Could you check a few things on this drawing? It's one solid part, dimensions in mm from its lowest x, y, z. A direction names the side the tool comes from. Round coordinates to 2 decimals unless told otherwise and drop trailing zeros. Write each loop counter-clockwise with the first axis right and the second up, starting at its lowest first coordinate (ties: lowest second). Pieces come first, ordered by that corner, then holes. Notation, with made-up numbers: (78.25, 71) - (104.25, 71) arc R33 ccw to (104.25, 105) - close; hole circle Ø5 at (-37.5, -39). An arc over 180 degrees is marked (long way). Use one line per item in the form item = value. Start each with the question number.
1. Which directions (+Z, -Z, +X, -X, +Y, -Y) give clear straight access to the entire face, cutting with the end or side of a thin tool? Please do the marked faces 4 and 5.
2. I want a section at A-A, the plane x = 10. List the corners of the cut face in (y, z) for me, plus the area to 3 significant figures.
3. We'd pull the mould along X, two halves only. Please class the marked faces 1, 2 and 3: +X half, -X half, draft (parallel to the pull), parting line (faces both ways), or undercut.
4. If I drill on line 1 along Y through (x, z) = (10, 5.75); line 2 along Z through (x, y) = (14.25, 14.5); line 3 along Y through (x, z) = (11.5, 1.25), over which ranges is the centre line in solid material (lowest first)?
5. Will this pin go through, and if not, where does the flat tip stop? pin 1 (2 mm diameter, centred on x = 7, z = 1, fed in from +Y).
6. I want a section at C-C, the plane z = 7. List the corners of the cut face in (x, y) for me, plus the area to 3 significant figures.
7. I want a section at B-B, the plane y = 4. List the corners of the cut face in (x, z) for me, plus the area to 3 significant figures.
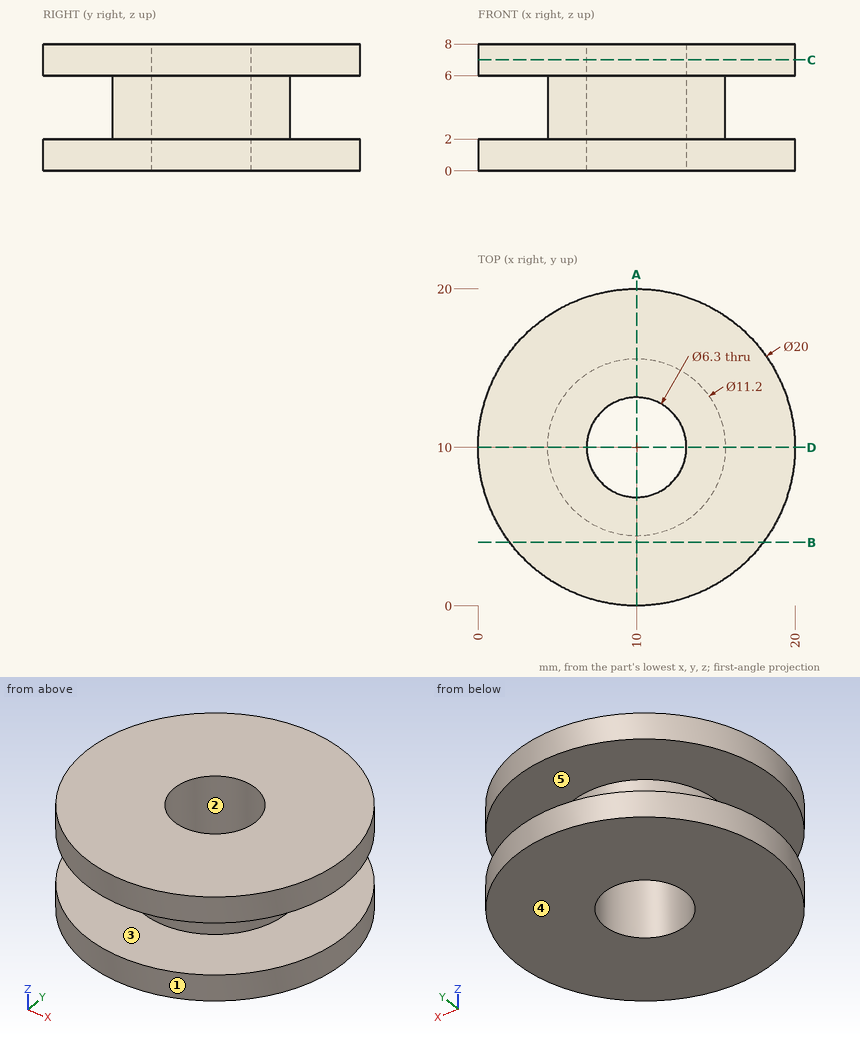
Model answer:
q1.face_4 = -Z, +X, -X, +Y, -Y
q1.face_5 = none
q2.outline = (0, 0) - (6.85, 0) - (6.85, 8) - (0, 8) - (0, 6) - (4.4, 6) - (4.4, 2) - (0, 2) - close; (13.15, 0) - (20, 0) - (20, 2) - (15.6, 2) - (15.6, 6) - (20, 6) - (20, 8) - (13.15, 8) - close
q2.area = 74.4 mm2
q3.face_1 = parting line
q3.face_2 = undercut
q3.face_3 = draft
q4.line_1 = 4.4 to 6.85, 13.15 to 15.6
q4.line_2 = 0 to 2, 6 to 8
q4.line_3 = 0.11 to 7.23, 12.77 to 19.89
q5.pin_1 = 19.8
q6.outline = circle Ø20 at (10, 10); hole circle Ø6.3 at (10, 10)
q6.area = 283 mm2
q7.outline = (2, 0) - (18, 0) - (18, 2) - (2, 2) - close; (2, 6) - (18, 6) - (18, 8) - (2, 8) - close
q7.area = 64.0 mm2
